Job drawing, mm, ordinate dimensions from the low corner. One solid piece. A direction names the side the tool comes from. Give positions to 0.01 mm unless a question says otherwise; leave off trailing zeros. Order: outer loops, then holes, each group sorted by start corner. A loop starts at its lowest first (then second) coordinate and runs counter-clockwise, first axis right, second up.
1. Probe line 1 (X direction, y = 10.5, z = 6.5); line 2 (Z direction, x = 22, y = 20.5); line 3 (Y direction, x = 38, z = 3). List the from-to ranges inside material, lowest first.
2. Mould opens along X. For the marked faces 5, 6 and 7 say: +X half, -X half, draft (parallel to the pull), parting line (faces both ways), or undercut.
3. Which spindle directions (+Z, -Z, +X, -X, +Y, -Y) get a long thin tool onto all of the face, cutting with end or side? Do the marked faces 1, 2, 3 and 4. Say none if no direction does.
4. Slice it at A-A on y = 25. List the corners of the cut face in (x, z), and give its area (3 significant figures).
5. Drop flat-ended pins along their axis: pin 1 Ø8 at (x, z) = (37, 10.5) entering from +Y; pin 2 Ø12 at (x, y) = (28, 4.5) entering from -Z; pin 3 Ø4 at (y, z) = (23.5, 18) entering from -X; pin 4 Ø10.5 at (y, z) = (23.5, 22.5) entering from +X. Give the stop position or say it passes through.
6. Slice it at B-B on z = 6.25. List the corners of the cut face in (x, y).
7. Slice it at C-C on x = 5.5. List the corners of the cut face in (y, z), and give its area (3 significant figures).
8. Slice it at D-D on y = 6. List the corners of the cut face in (x, z), and give its area (3 significant figures).
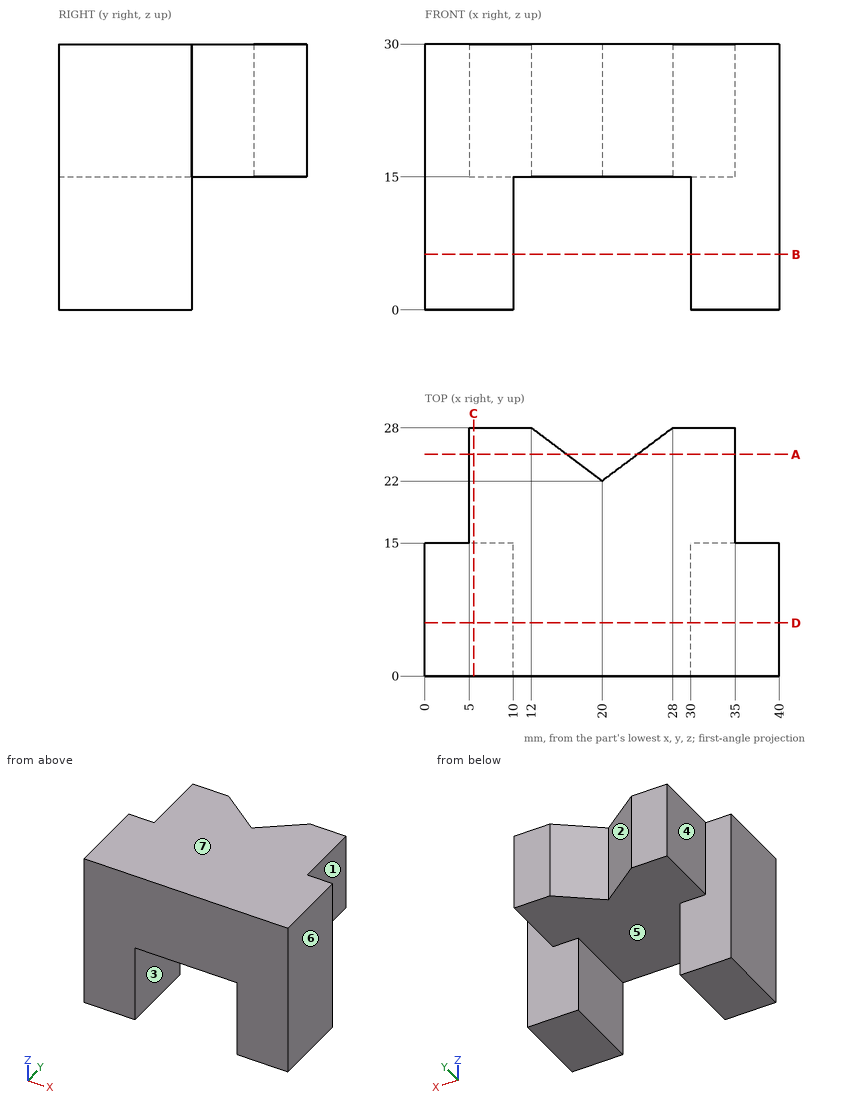
Data:
1. line 1: x = 0 to 10, 30 to 40
1. line 2: z = 15 to 30
1. line 3: y = 0 to 15
2. face 5: undercut
2. face 6: +X half
2. face 7: draft
3. face 1: +Z, -Z, +X, +Y
3. face 2: +Z, -Z, +Y
3. face 3: -Z, +Y, -Y
3. face 4: +Z, -Z, -X, +Y
4. outline: (5, 15) - (16, 15) - (16, 30) - (5, 30) - close; (24, 15) - (35, 15) - (35, 30) - (24, 30) - close
4. area: 330 mm2
5. pin 1: stops at y = 15
5. pin 2: stops at z = 0
5. pin 3: stops at x = 5
5. pin 4: stops at x = 35
6. outline: (0, 0) - (10, 0) - (10, 15) - (0, 15) - close; (30, 0) - (40, 0) - (40, 15) - (30, 15) - close
7. outline: (0, 0) - (15, 0) - (15, 15) - (28, 15) - (28, 30) - (0, 30) - close
7. area: 645 mm2
8. outline: (0, 0) - (10, 0) - (10, 15) - (30, 15) - (30, 0) - (40, 0) - (40, 30) - (0, 30) - close
8. area: 900 mm2
